Autodesk Inventor part; units mm, degrees
ref_plane "YZ Plane" through (0, 0, 0) normal (1, 0, 0) x (0, 1, 0)
ref_plane "XZ Plane" through (0, 0, 0) normal (0, 1, 0) x (-1, 0, 0)
ref_plane "XY Plane" through (0, 0, 0) normal (0, 0, 1) x (1, 0, 0)
sketch "Sketch1" plane through (0, 0, 0) normal (0, 1, 0) x (-1, 0, 0)
  line L0 (0, 0) -> (-12.77, 0)
  line L1 (-12.77, 0) -> (-12.77, 6.9)
  line L2 (-12.77, 6.9) -> (0, 6.9)
  line L3 (0, 6.9) -> (0, 0)
  line L4 (3, -3) -> (-15.77, -3)
  line L5 (-15.77, -3) -> (-15.77, 9.9)
  line L6 (-15.77, 9.9) -> (3, 9.9)
  line L7 (3, 9.9) -> (3, -3)
  point P0 (-6.385, -3)
  point P1 (-6.385, 0)
  point P2 (3, 3.45)
  dimension "d0" = 12.77
  dimension "d1" = 6.9
  dimension "d2" = 3
  dimension "d3" = 3
  dimension "d4" = 3
  dimension "d5" = 3
extrude "Extrusion1" add sketch "Sketch1" along normal blind 8.8
sketch "Sketch2" plane through (0, 0, 0) normal (0, -1, 0) x (1, 0, 0)
  line L0 (-3, 9.9) -> (15.77, 9.9)
  line L1 (15.77, -3) -> (-3, -3)
  line L2 (-3, 9.9) -> (15.77, 9.9)
  line L3 (15.77, 9.9) -> (15.77, -3)
  line L4 (15.77, -3) -> (-3, -3)
  line L5 (-3, -3) -> (-3, 9.9)
  point P0 (0, 0)
extrude "Extrusion2" add sketch "Sketch2" along normal blind 3
sketch "Sketch3" plane through (0, 0, 0) normal (0, 1, 0) x (1, 0, 0)
  line L0 (0, -6.9) -> (0, 0)
  line L1 (12.77, -6.9) -> (0, -6.9)
  line L2 (0, 0) -> (8.3, 0)
  line L3 (8.3, 0) -> (8.3, -6.9)
  line L4 (8.3, -6.9) -> (0, -6.9)
  line L5 (0, -6.9) -> (0, 0)
  dimension "d10" = 8.3
extrude "Extrusion3" cut sketch "Sketch3" against normal blind 3
equation "\"d3\" = d2"
equation "\"d5\" = d4"
properties part number "switch test v01"
Model file for the job. Use its own axes, mm. A direction names the side the tool comes from. Coordinates: 2 decimals unless noted, no trailing zeros. Loops run counter-clockwise (first coordinate to the right, second up) from the corner with the lowest first, then second, coordinate; pieces in that order, holes last. Notation, with made-up numbers: (30, -11) - (47, -11) arc R26 cw to (47, 24) - close; hole circle Ø7 at (36.5, 37.25). An arc over 180 degrees is marked (long way). Write item = value, one per line. Start each with the question number.
Item 1: 3-axis set-ups, long thin cutter, end or side, ignore diameter. For faces 1 (the face through (12.77, 4, 3)), 2 (the face through (0, 3, 3)), 3 (the face through (7, 3, 9.9)): which of +Z, -Z, +X, -X, +Y, -Y reach the whole face in a straight line?
Item 2: Saw through at C-C, the plane x = 7.5. List the corners of the cut face in (y, z), then the cut area to 3 significant figures.
Item 3: Drop a flat-ended pin along its axis: pin 1 Ø2 at (x, z) = (10.5, 4) entering from +Y. Give the stop position or say it passes through.
Item 4: Pull direction X, two halves, no side cores. Call faces 4 (the face through (11, 0, 3)), 5 (the face through (15.77, 3, 3)), 6 (the face through (6, 3, -3)): +X half, -X half, draft (parallel to the pull), parting line (faces both ways), or undercut.
Item 5: Saw through at B-B, the plane y = -1. List the corners of the cut face in (x, z), then the cut area to 3 significant figures.
Item 6: Saw through at D-D, the plane y = 4.5. List the corners of the cut face in (x, z), then the cut area to 3 significant figures.
Item 7: Wall check: probe 1 along X at (y, z) = (2.75, 6.25); probe 2 along Z at (x, y) = (3.75, -1.75); probe 3 along X at (y, z) = (-1, 3.5). Give the ranges that are in metal, low to high. Write a range as [from, to].
Item 8: Saw through at A-A, the plane z = 0.75. List the corners of the cut face in (x, y).
Answers:
q1.face_1 = +Y
q1.face_2 = +Y, -Y
q1.face_3 = +Z, +X, -X, +Y, -Y
q2.outline = (-3, -3) - (8.8, -3) - (8.8, 0) - (-3, 0) - close; (-3, 6.9) - (8.8, 6.9) - (8.8, 9.9) - (-3, 9.9) - close
q2.area = 70.8 mm2
q3.pin_1 = 0
q4.face_4 = undercut
q4.face_5 = +X half
q4.face_6 = draft
q5.outline = (-3, -3) - (15.77, -3) - (15.77, 9.9) - (-3, 9.9) - close; hole (0, 0) - (8.3, 0) - (8.3, 6.9) - (0, 6.9) - close
q5.area = 185 mm2
q6.outline = (-3, -3) - (15.77, -3) - (15.77, 9.9) - (-3, 9.9) - close; hole (0, 0) - (12.77, 0) - (12.77, 6.9) - (0, 6.9) - close
q6.area = 154 mm2
q7.probe_1 = [-3, 0], [12.77, 15.77]
q7.probe_2 = [-3, 0], [6.9, 9.9]
q7.probe_3 = [-3, 0], [8.3, 15.77]
q8.outline = (-3, -3) - (0, -3) - (0, 8.8) - (-3, 8.8) - close; (8.3, -3) - (15.77, -3) - (15.77, 8.8) - (12.77, 8.8) - (12.77, 0) - (8.3, 0) - close
